Autodesk Inventor part; units mm, degrees
ref_plane "YZ Plane" through (0, 0, 0) normal (1, 0, 0) x (0, 1, 0)
ref_plane "XZ Plane" through (0, 0, 0) normal (0, 1, 0) x (-1, 0, 0)
ref_plane "XY Plane" through (0, 0, 0) normal (0, 0, 1) x (1, 0, 0)
sketch "Sketch1" plane through (0, 0, 0) normal (0, 0, 1) x (1, 0, 0)
  circle A0 centre (0, 0) radius 25
  dimension "d0" = 50
extrude "Extrusion1" add sketch "Sketch1" along normal blind 4
sketch "Sketch2" plane through (0, 0, 4) normal (0, 0, 1) x (1, 0, 0)
  circle A0 centre (0, 15) radius 1.5
  line L0 (0, -35) -> (0, 35)
  point P0 (0, 0)
  dimension "d3" = 3
  dimension "d4" = 15
extrude "Extrusion2" cut sketch "Sketch2" against normal blind 10
pattern_circular "Circular Pattern1" count 6 over 360 about axis through (0, 0, -10) along (0, 0, 1) of "Extrusion2"
sketch "Sketch3" plane through (0, 0, 4) normal (0, 0, 1) x (1, 0, 0)
  circle A0 centre (0, 0) radius 4.5
  dimension "d11" = 9
extrude "Extrusion3" cut sketch "Sketch3" against normal blind 10
properties part number "center_cover2"
Design review of the part built by this model. Coordinates are the model's own, in mm. Round coordinates to 2 decimals unless told otherwise and drop trailing zeros. Order: outer loops, then holes, each group sorted by start corner. A loop starts at its lowest first (then second) coordinate and runs counter-clockwise, first axis right, second up. Notation, with made-up numbers: (30.5, -11.75) - (89.5, -11.75) arc R23 cw to (89.5, 12.25) - close; hole circle Ø6 at (60.25, -38.75). An arc over 180 degrees is marked (long way). One line per question, with ' | ' between items.
Item 1: Take a section at D-D, the plane x = -7. Write out the cut boundary in (y, z), then the cut area to 3 significant figures.
Checks:
outline: (-24, 0) - (24, 0) - (24, 4) - (-24, 4) - close | area: 192 mm²
Item 2: For P1, Ø3.5, axis at x = -12.99, y = 7.5, coming from the +Z side; P2, Ø2, axis at x = 12, z = 0.5, coming from the -Y side; P3, Ø1.5, axis at x = 0, z = 2, coming from the -Y side; P4, Ø1.5, axis at x = -14, z = 2, coming from the +Y side, all flat-tipped, find the tip position at first contact; note any pin that passes through.
Checks:
P1: z = 4 | P2: y = -22.45 | P3: y = -25 | P4: y = 21.2
Item 3: Wall thickness on line 1 (Y direction, x = 0, z = 2.4); line 2 (X direction, y = -8, z = 0.6); line 3 (X direction, y = 7, z = 0.5): over which ranges is each line inside the solid? List them lowest first. Write a range as [from, to].
Checks:
line 1: [-25, -16.5], [-13.5, -4.5], [4.5, 13.5], [16.5, 25] | line 2: [-23.69, -14.4], [-11.58, 11.58], [14.4, 23.69] | line 3: [-24, -14.4], [-11.58, 11.58], [14.4, 24]
Item 4: Take a section at B-B, the plane z = 1.75. Write out the cut boundary in (x, y), then the cut area to 3 significant figures.
Checks:
outline: circle Ø50 at (0, 0); hole circle Ø3 at (-12.99, -7.5); hole circle Ø3 at (-12.99, 7.5); hole circle Ø9 at (0, 0); hole circle Ø3 at (0, -15); hole circle Ø3 at (0, 15); hole circle Ø3 at (12.99, -7.5); hole circle Ø3 at (12.99, 7.5) | area: 1,860 mm²
Item 5: Draft analysis for pull direction X (two halves, no side actions). For faces 1 (the face through (1.11, -16.01, 2.03)), 2 (the face through (23.846, -7.509, 1.972)), 3 (the face through (5, 0, 0)), 4 (the face through (11.8, -8.41, 2.03)), state which applies: +X half, -X half, draft (parallel to the pull), parting line (faces both ways), or undercut.
Checks:
face 1: undercut | face 2: parting line | face 3: draft | face 4: undercut
Item 6: Take a section at A-A, the plane y = 15. Write out the cut boundary in (x, z), then the cut area to 3 significant figures.
Checks:
outline: (-20, 0) - (-1.5, 0) - (-1.5, 4) - (-20, 4) - close; (1.5, 0) - (20, 0) - (20, 4) - (1.5, 4) - close | area: 148 mm²
Item 7: Take a section at C-C, the plane y = 7. Write out the cut boundary in (x, z), then the cut area to 3 significant figures.
Checks:
outline: (-24, 0) - (-14.4, 0) - (-14.4, 4) - (-24, 4) - close; (-11.58, 0) - (11.58, 0) - (11.58, 4) - (-11.58, 4) - close; (14.4, 0) - (24, 0) - (24, 4) - (14.4, 4) - close | area: 169 mm²
